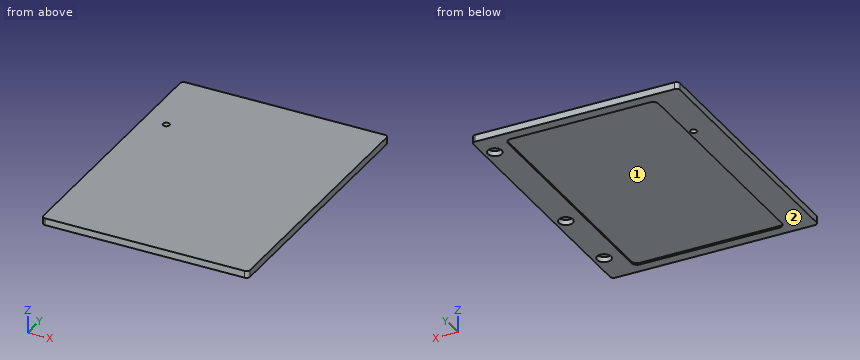
```python
from build123d import *

# Parameters (mm, degrees)
SKETCH_1_W               = 591
SKETCH_1_H               = 770
EXTRUDE_1_DEPTH          = 20
CUT_EXTRUDE_1_DEPTH      = 825.997121207
CUT_EXTRUDE_1_DEPTH_BACK = 825.997121207
SKETCH_2_R               = 9.1
FILLET_1_R               = 10
SKETCH_4_R               = 20.1
CUT_EXTRUDE_3_DEPTH      = 15
SKETCH_5_W               = 431
SKETCH_5_H               = 710
CUT_EXTRUDE_4_DEPTH      = 5
FILLET_2_R               = 16


with BuildPart() as part:
    # 草图1 → 凸台-拉伸1 (new body)
    with BuildSketch(Plane.XY):
        with Locations((0, 385)):
            Rectangle(SKETCH_1_W, SKETCH_1_H)
    extrude(amount=EXTRUDE_1_DEPTH)

    # 草图2 → 切除-拉伸1 (cut, two sides: drawn at the far end of the back side and taken through both)
    with BuildSketch(Plane.XY.offset(20).offset(-CUT_EXTRUDE_1_DEPTH_BACK)):
        with Locations((-230.5, 560)):
            Circle(SKETCH_2_R)
    extrude(amount=CUT_EXTRUDE_1_DEPTH + CUT_EXTRUDE_1_DEPTH_BACK, mode=Mode.SUBTRACT)

    # 圆角1
    fillet_1_edges = [part.edges().sort_by_distance(p)[0] for p in [
        (-295.5, 770, 10),
        (295.5, 770, 10),
        (295.5, 0, 10),
        (-295.5, 0, 10),
    ]]
    fillet(fillet_1_edges, radius=FILLET_1_R)

    # 草图4 → 切除-拉伸3 (cut)
    with BuildSketch(Plane(origin=(0, 0, 0), x_dir=(-1, 0, 0), z_dir=(0, 0, -1))):
        with Locations((-265.5, 700)):
            Circle(SKETCH_4_R)
        with Locations((-265.5, 310)):
            Circle(SKETCH_4_R)
        with Locations((-265.5, 100)):
            Circle(SKETCH_4_R)
    extrude(amount=-CUT_EXTRUDE_3_DEPTH, mode=Mode.SUBTRACT)

    # 草图5 → 切除-拉伸4 (cut)
    with BuildSketch(Plane(origin=(0, 0, 0), x_dir=(-1, 0, 0), z_dir=(0, 0, -1))):
        with Locations((0, 385)):
            Rectangle(SKETCH_5_W, SKETCH_5_H)
    extrude(amount=-CUT_EXTRUDE_4_DEPTH, mode=Mode.SUBTRACT)

    # 圆角2
    fillet_2_edges = [part.edges().sort_by_distance(p)[0] for p in [
        (215.5, 30, 2.5),
        (215.5, 740, 2.5),
        (-215.5, 740, 2.5),
        (-215.5, 30, 2.5),
    ]]
    fillet(fillet_2_edges, radius=FILLET_2_R)


solid = part.part
```
Build history of the part. All positions in model axes, mm. Face numbers are marked on the shaded views. Coordinates: 2 decimals unless noted, no trailing zeros. Order: outer loops, then holes, each group sorted by start corner. A loop starts at its lowest first (then second) coordinate and runs counter-clockwise, first axis right, second up. Notation, with made-up numbers: (82.25, 56) -> (127.25, 56) arc R35 cw to (127.25, 94) -> close; hole circle Ø1 at (38.25, 63). An arc over 180 degrees is marked (long way). Answer in a Markdown table with one row per item. Add a question column.
Q1. Drop flat-ended pins along their axis: pin 1 (12 mm diameter, centred on x = 268.5, y = 320, fed in from -Z); pin 2 (6 mm diameter, centred on x = -44, y = 415, fed in from -Z). Give the stop position or say it passes through.
Q2. Mould opens along Y. For the marked faces 1 and 2 say: +Y half, -Y half, draft (parallel to the pull), parting line (faces both ways), or undercut.
Q3. Band-saw the part on B-B, the plane y = 560. List the corners of the cut face in (x, z), then the cut area to 3 significant figures.
Q4. Band-saw the part on C-C, the plane x = -14. List the corners of the cut face in (y, z).
Q5. Band-saw the part on A-A, the plane x = -230.5. List the corners of the cut face in (y, z).
Q6. Band-saw the part on D-D, the plane y = 201.5. List the corners of the cut face in (x, z), then the cut area to 4 significant figures.
Q7. Wall check: line 1 along Y through (x, z) = (265.5, 8.75); line 2 along Y through (x, z) = (267, 6); line 3 along Y through (x, z) = (-230.5, 14.5). Give the ranges that are in metal, low to high. Write a range as [from, to].
Answers follow:
| question | item | result |
|---|---|---|
| 1 | pin 1 | z = 15 |
| 1 | pin 2 | z = 5 |
| 2 | face 1 | undercut |
| 2 | face 2 | draft |
| 3 | outline | (-295.5, 0) -> (-239.6, 0) -> (-239.6, 20) -> (-295.5, 20) -> close; (-221.4, 0) -> (-215.5, 0) -> (-215.5, 5) -> (215.5, 5) -> (215.5, 0) -> (295.5, 0) -> (295.5, 20) -> (-221.4, 20) -> close |
| 3 | area | 9,300 mm^2 |
| 4 | outline | (0, 0) -> (30, 0) -> (30, 5) -> (740, 5) -> (740, 0) -> (770, 0) -> (770, 20) -> (0, 20) -> close |
| 5 | outline | (0, 0) -> (550.9, 0) -> (550.9, 20) -> (0, 20) -> close; (569.1, 0) -> (770, 0) -> (770, 20) -> (569.1, 20) -> close |
| 6 | outline | (-295.5, 0) -> (-215.5, 0) -> (-215.5, 5) -> (215.5, 5) -> (215.5, 0) -> (295.5, 0) -> (295.5, 20) -> (-295.5, 20) -> close |
| 6 | area | 9,665 mm^2 |
| 7 | line 1 | [0, 79.9], [120.1, 289.9], [330.1, 679.9], [720.1, 770] |
| 7 | line 2 | [0, 79.96], [120.04, 289.96], [330.04, 679.96], [720.04, 770] |
| 7 | line 3 | [0, 550.9], [569.1, 770] |
